Autodesk Inventor part; units mm, degrees
ref_plane "YZ Plane" through (0, 0, 0) normal (1, 0, 0) x (0, 1, 0)
ref_plane "XZ Plane" through (0, 0, 0) normal (0, 1, 0) x (-1, 0, 0)
ref_plane "XY Plane" through (0, 0, 0) normal (0, 0, 1) x (1, 0, 0)
sketch "Esquisse1" plane through (0, 0, 0) normal (0, 1, 0) x (-1, 0, 0)
  circle A0 centre (0, 0) radius 5 construction
  circle A1 centre (0, 0) radius 120
  dimension "d0" = 10
  dimension "d39" = 240
extrude "Extrusion1" add sketch "Esquisse1" along normal blind 5
sketch "Esquisse2" plane through (0, 5, 0) normal (0, 1, 0) x (1, 0, 0)
  circle A0 centre (0, 0) radius 5
  dimension "d5" = 10
extrude "Extrusion2" cut sketch "Esquisse2" against normal up to surface (5 mm away)
sketch "Esquisse3" plane through (0, 0, 0) normal (0, -1, 0) x (1, 0, 0)
  circle A0 centre (0, 0) radius 5
  circle A1 centre (0, 0) radius 12.5
  dimension "d8" = 25
extrude "Extrusion3" cut sketch "Esquisse3" against normal blind 2
chamfer "Chanfrein1" distance 0.5 angle 45 3 edges at (-12.5, 0, 0) (-5, 2, 0) (-5, 5, 0)
sketch "Esquisse4" plane through (0, 5, 0) normal (0, 1, 0) x (1, 0, 0)
  point P0 (0, 0)
  point P1 (0, -30)
  point P2 (25.9808, 15)
  point P3 (-25.9808, 15)
  dimension "d14" = 30
  dimension "d17" = 360
hole "Perçage1" at (0, 5, 30) at (25.9808, 5, -15) at (-25.9808, 5, -15) direction (0, -1, 0) diameter 4.2 depth 3 tip angle 118
sketch "Esquisse6" plane through (0, 5, 0) normal (0, 1, 0) x (1, 0, 0)
  circle A0 centre (-107, 0) radius 3
  point P0 (0, 0)
  dimension "d42" = 6
  dimension "d43" = 107
extrude "Extrusion5" cut sketch "Esquisse6" against normal up to surface (5 mm away)
properties part number "tourelle"
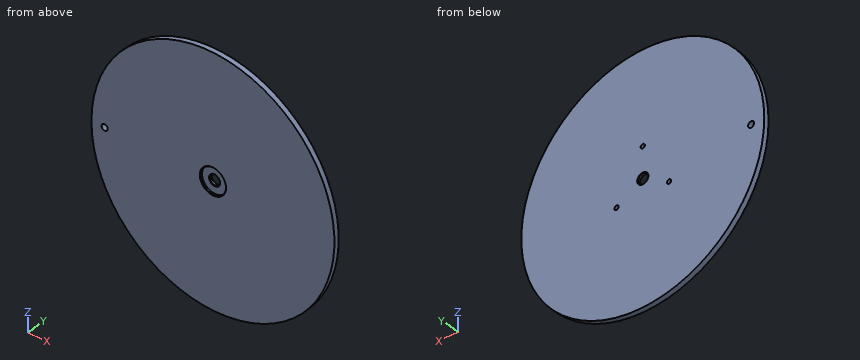
Here's how the part is built. I have some questions about the finished solid (model axes, mm). Give positions to 0.01 mm unless a question says otherwise; leave off trailing zeros. Write each loop counter-clockwise with the first axis right and the second up, starting at its lowest first coordinate (ties: lowest second). Pieces come first, ordered by that corner, then holes. Notation, with made-up numbers: (-1, 40.25) -> (43, 40.25) arc R22 ccw to (43, 79.25) -> close; hole circle Ø7 at (47.25, -11). An arc over 180 degrees is marked (long way). Write each question's results on one line, items separated by ' | '.
Item 1: If I drill on L1, parallel to X at y = 4.15, z = -15; L2, parallel to X at y = 2.1, z = -16; L3, parallel to Z at x = 9, y = 0.85, over which ranges is the centre line in solid material (lowest first)?
Output:
L1: x = -119.06 to -28.08, -23.88 to 23.88, 28.08 to 119.06 | L2: x = -118.93 to -27.83, -24.13 to 24.13, 27.83 to 118.93 | L3: z = -119.66 to -8.67, 8.67 to 119.66
Item 2: Suppose I cut it at B-B on z = 0. Write out the boundary of the cut face in (x, y).
Output:
outline: (-120, 0) -> (-110, 0) -> (-110, 5) -> (-120, 5) -> close; (-104, 0) -> (-13, 0) -> (-12.5, 0.5) -> (-12.5, 2) -> (-5.5, 2) -> (-5, 2.5) -> (-5, 4.5) -> (-5.5, 5) -> (-104, 5) -> close; (5, 2.5) -> (5.5, 2) -> (12.5, 2) -> (12.5, 0.5) -> (13, 0) -> (120, 0) -> (120, 5) -> (5.5, 5) -> (5, 4.5) -> close
Item 3: Suppose I cut it at D-D on z = 57.5. Write out the boundary of the cut face in (x, y).
Output:
outline: (-105.33, 0) -> (105.33, 0) -> (105.33, 5) -> (-105.33, 5) -> close
Item 4: Suppose I cut it at A-A on x = -107. Write out the boundary of the cut face in (y, z), plus the area to 3 significant figures.
Output:
outline: (0, -54.32) -> (5, -54.32) -> (5, -3) -> (0, -3) -> close; (0, 3) -> (5, 3) -> (5, 54.32) -> (0, 54.32) -> close | area: 513 mm^2
Item 5: For pin 1 Ø3 at (x, y) = (-34.5, 0.5) entering from -Z; pin 2 Ø1.5 at (y, z) = (4.5, 4.5) entering from +X; pin 3 Ø2 at (y, z) = (4, 46) entering from -X, each with a flat end and sliding along its axis, tell me the tip position at first contact or that it passes through.
Output:
pin 1: stops at z = -115.37 | pin 2: stops at x = 119.94 | pin 3: stops at x = -111.24
Item 6: Suppose I cut it at C-C on x = -48. Write out the boundary of the cut face in (y, z).
Output:
outline: (0, -109.98) -> (5, -109.98) -> (5, 109.98) -> (0, 109.98) -> close
